Check sheet for the modelled part. Datum: model origin and axes. Units: mm. A direction names the side the tool comes from. Round coordinates to 2 decimals unless told otherwise and drop trailing zeros. Write each loop counter-clockwise with the first axis right and the second up, starting at its lowest first coordinate (ties: lowest second). Pieces come first, ordered by that corner, then holes. Notation, with made-up numbers: M -29.5,-16 L -1.5,-16 A20 cw -1.5,-3 Z; hole C 68.25,37.25 d1. An arc over 180 degrees is marked long. Put each result on its own line as item: value.
Autodesk Inventor part; units mm, degrees
ref_plane "YZ Plane" through (0, 0, 0) normal (1, 0, 0) x (0, 1, 0)
ref_plane "XZ Plane" through (0, 0, 0) normal (0, 1, 0) x (-1, 0, 0)
ref_plane "XY Plane" through (0, 0, 0) normal (0, 0, 1) x (1, 0, 0)
sketch "Эскиз1" plane through (0, 0, 0) normal (0, 0, 1) x (1, 0, 0)
  line L0 (0, 0) -> (44.5, 0)
  line L1 (44.5, 0) -> (44.5, 35.5)
  line L2 (44.5, 35.5) -> (0, 35.5)
  line L3 (0, 35.5) -> (0, 0)
  dimension "d0" = 44.5
  dimension "d1" = 35.5
extrude "Выдавливание1" add sketch "Эскиз1" along normal blind 1.7
sketch "Эскиз2" plane through (0, 0, 1.7) normal (0, 0, 1) x (1, 0, 0)
  line L0 (0, 0) -> (44.5, 0)
  line L1 (44.5, 0) -> (44.5, 3.5)
  line L2 (44.5, 0) -> (44.5, 35.5)
  line L3 (44.5, 3.5) -> (41, 3.5)
  line L4 (44.5, 35.5) -> (44.5, 32)
  line L5 (44.5, 32) -> (41, 32)
  line L6 (44.5, 35.5) -> (0, 35.5)
  point P0 (36, 33)
  point P1 (36, 2.5)
  point P2 (36, 33)
  dimension "d4" = 3.5
  dimension "d5" = 3.5
  dimension "d6" = 3.5
  dimension "d7" = 3.5
  dimension "d26" = 8.5
  dimension "d27" = 8.5
  dimension "d28" = 2.5
  dimension "d29" = 2.5
hole "Отверстие1" at (41, 32, 1.7) at (41, 3.5, 1.7) at (36, 33, 1.7) at (36, 2.5, 1.7) direction (0, 0, -1) diameter 3.35 depth 15
sketch "Эскиз3" plane through (0, 0, 0) normal (0, 0, -1) x (-1, 0, 0)
  line L0 (-44.5, 0) -> (-44.5, 35.5)
  line L1 (-44.5, 0) -> (-44.5, 9.25)
  line L2 (-44.5, 9.25) -> (-27.5, 9.25)
  line L3 (-27.5, 9.25) -> (-27.5, 26.25)
  line L4 (-27.5, 26.25) -> (-44.5, 26.25)
  line L5 (-44.5, 26.25) -> (-44.5, 9.25)
  line L6 (-36, 26.25) -> (-36, 27.75)
  line L7 (-36, 9.25) -> (-36, 7.75)
  circle A0 centre (-36, 7.75) radius 2.5
  circle A1 centre (-36, 27.75) radius 2.5
  line L8 (-38.5, 27.75) -> (-33.5, 27.75)
  line L9 (-33.5, 27.75) -> (-33.5, 26.25)
  line L10 (-33.5, 26.25) -> (-38.5, 26.25)
  line L11 (-38.5, 26.25) -> (-38.5, 27.75)
  line L12 (-33.5, 7.75) -> (-38.5, 7.75)
  line L13 (-38.5, 7.75) -> (-38.5, 9.25)
  line L14 (-38.5, 9.25) -> (-33.5, 9.25)
  line L15 (-33.5, 9.25) -> (-33.5, 7.75)
  point P0 (0, 0)
  dimension "d20" = 5
  dimension "d21" = 5
  dimension "d15" = 9.25
  dimension "d16" = 17
  dimension "d17" = 17
  dimension "d18" = 1.5
  dimension "d19" = 1.5
extrude "Выдавливание2" add sketch "Эскиз3" along normal blind 8
sketch "Эскиз4" plane through (0, 0, -8) normal (0, 0, -1) x (-1, 0, 0)
  line L0 (-44.5, 0) -> (-44.5, 35.5)
  line L1 (-44.5, 17.75) -> (-27.5, 17.75)
  line L2 (-27.5, 26.25) -> (-27.5, 9.25)
  circle A0 centre (-36, 17.75) radius 8.5
  point P0 (0, 0)
extrude "Выдавливание3" add sketch "Эскиз4" along normal blind 14
equation "\"d4\" = d6"
equation "\"d5\" = d6"
equation "\"d7\" = d6"
properties part number "Техническое зрение OpenMV"
1. Release check for a two-part mould opening along Y. For faces 1 (the flat face through (44.5, 18, -2)), 2 (the flat face through (42, 9.25, -4)), 3 (the cylindrical face through (34.34, 33.22, 0.84)) record: +Y half, -Y half, draft (parallel to the pull), parting line (faces both ways), or undercut.
Computed values:
face 1: draft
face 2: -Y half
face 3: undercut
2. Cross-section at D-D (y = 29). Enter the section's corners in (x, z), then the cut area to 3 significant figures.
Computed values:
outline: M 0,0 L 33.83,0 L 33.83,-8 L 38.17,-8 L 38.17,0 L 44.5,0 L 44.5,1.7 L 0,1.7 Z
area: 110 mm2
3. Access from +Z, -Z, +X, -X, +Y, -Y to the whole of each face (thin tool, end or side, straight path). Record for faces 4 (the flat face through (38.5, 8, -4)), 5 (the flat face through (31, 9.25, -4)), 6 (the flat face through (34.78, 26.34, -8)), 7 (the flat face through (41, 26.25, -4)).
Computed values:
face 4: -Z, +X, -Y
face 5: -Z, -X, -Y
face 6: -Z, +Y
face 7: -Z, +X, +Y
4. Scan lines: probe 1 along Y at (x, z) = (41, 1.25) (3 decimals); probe 2 along Y at (x, z) = (36, 1.3) (3 decimals); probe 3 along X at (y, z) = (3.5, 0.9) (3 decimals). Record each from-to range of solid material in increasing order.
Computed values:
probe 1: y = 0 to 1.825, 5.175 to 30.325, 33.675 to 35.5
probe 2: y = 0 to 0.825, 4.175 to 31.325, 34.675 to 35.5
probe 3: x = 0 to 34.656, 37.344 to 39.325, 42.675 to 44.5
5. Cross-section at A-A (x = 36). Enter the section's corners in (y, z) (3 decimals).
Computed values:
outline: M 0,0 L 0.825,0 L 0.825,1.7 L 0,1.7 Z; M 4.175,0 L 5.25,0 L 5.25,-8 L 9.25,-8 L 9.25,-22 L 26.25,-22 L 26.25,-8 L 30.25,-8 L 30.25,0 L 31.325,0 L 31.325,1.7 L 4.175,1.7 Z; M 34.675,0 L 35.5,0 L 35.5,1.7 L 34.675,1.7 Z
6. Cross-section at C-C (z = -16.25). Enter the section's corners in (x, y), then the cut area to 3 significant figures.
Computed values:
outline: C 36,17.75 d17
area: 227 mm2
7. Depth check by flat-ended pin: pin 1 Ø1.8 at (x, z) = (40.5, -2.5) entering from +Y; pin 2 Ø6.5 at (x, z) = (41, -5.5) entering from -Y; pin 3 Ø10 at (y, z) = (30.5, -11.5) entering from -X. Enter the tip coordinate at first touch or a pass-through.
Computed values:
pin 1: stops at y = 26.25
pin 2: stops at y = 5.96
pin 3: stops at x = 32.51
8. Cross-section at B-B (y = 33). Enter the section's corners in (x, z) (3 decimals), then the cut area to 3 significant figures.
Computed values:
outline: M 0,0 L 34.325,0 L 34.325,1.7 L 0,1.7 Z; M 37.675,0 L 39.656,0 L 39.656,1.7 L 37.675,1.7 Z; M 42.344,0 L 44.5,0 L 44.5,1.7 L 42.344,1.7 Z
area: 65.4 mm2
